from build123d import *

# Parameters (mm, degrees)
SKETCH1_R                  = 2
SCREW_SECTION_DEPTH        = 17
SKETCH2_R                  = 3.5
BAR_SECTION_DEPTH          = 24
MOUNT_SECTION_DEPTH        = 1.6
BAR_TAPER_DEPTH            = 6
MOUNT_FILLET_R             = 0.5
MOUNT_FILLET_OF_MIRROR_2_R = 0.5


with BuildPart() as part:
    # Sketch1 → Screw Section (new body)
    with BuildSketch(Plane.XY):
        Circle(SKETCH1_R)
    screw_section = extrude(amount=SCREW_SECTION_DEPTH)

    # Sketch2 → Bar Section (add)
    with BuildSketch(Plane.XY.offset(17)):
        Circle(SKETCH2_R)
    bar_section = extrude(amount=BAR_SECTION_DEPTH)

    # Sketch3 → Mount Section (add, symmetric)
    with BuildSketch(Plane(origin=(0, 0, 0), x_dir=(1, 0, 0), z_dir=(0, 1, 0))):
        with BuildLine():
            Line((5, -41), (-5, -41))
            Line((-5, -41), (-5, -46))
            ThreePointArc((-5, -46), (0, -51), (5, -46))
            Line((5, -46), (5, -41))
        make_face()
    mount_section = extrude(amount=MOUNT_SECTION_DEPTH, both=True)

    # Sketch4 → Bar Taper (cut, symmetric)
    with BuildSketch(Plane(origin=(0, 0, 0), x_dir=(0, 0, -1), z_dir=(1, 0, 0))):
        Polygon((-36, -3.5), (-41, -1.6), (-41, -3.5), align=None)
        Polygon((-36, 3.5), (-41, 1.6), (-41, 3.5), align=None)
    bar_taper = extrude(amount=BAR_TAPER_DEPTH, both=True, mode=Mode.SUBTRACT)

    # Mount Fillet
    mount_fillet_edges = [part.edges().sort_by_distance(p)[0] for p in [
        (-5, 0, 41),
        (3.401842713, -0.823083322, 41),
        (-3.5, 0, 41),
        (5, 0, 41),
    ]]
    fillet(mount_fillet_edges, radius=MOUNT_FILLET_R)

    # Sketch6 → Ball Hole (revolve, cut)
    with BuildSketch(Plane(origin=(0, 0, 0), x_dir=(0, 0, -1), z_dir=(1, 0, 0))):
        with BuildLine():
            Line((-47.920937271, -1.6), (-46, -1.6))
            Line((-46, -1.6), (-46, 1.6))
            Line((-46, 1.6), (-47.920937271, 1.6))
            ThreePointArc((-47.920937271, 1.6), (-48.5, 0), (-47.920937271, -1.6))
        make_face()
    ball_hole = revolve(axis=Axis((0, -1.6, 46), (0, 1, 0)), mode=Mode.SUBTRACT)

    # Mirror 2: Screw Section, Bar Section, Mount Section, Bar Taper, Ball Hole across Front Plane
    add(screw_section.mirror(Plane.XY))
    add(bar_section.mirror(Plane.XY))
    add(mount_section.mirror(Plane.XY))
    add(bar_taper.mirror(Plane.XY), mode=Mode.SUBTRACT)
    add(ball_hole.mirror(Plane.XY), mode=Mode.SUBTRACT)

    # Mount Fillet of Mirror 2
    mount_fillet_of_mirror_2_edges = [part.edges().sort_by_distance(p)[0] for p in [
        (-5, 0, -41),
        (3.401842713, -0.823083322, -41),
        (-3.5, 0, -41),
        (5, 0, -41),
    ]]
    fillet(mount_fillet_of_mirror_2_edges, radius=MOUNT_FILLET_OF_MIRROR_2_R)


solid = part.part
Geometry: final body of the model. Coordinates: model frame, mm. A direction names the side the tool comes from. Coordinates: 2 decimals unless noted, no trailing zeros. Write each loop counter-clockwise with the first axis right and the second up, starting at its lowest first coordinate (ties: lowest second). Pieces come first, ordered by that corner, then holes. Notation, with made-up numbers: (83.25, 50.5) - (135.25, 50.5) arc R33 cw to (135.25, 82.5) - close; hole circle Ø9 at (-21, -22). An arc over 180 degrees is marked (long way). Return JSON: item names as keys, results as strings.
Item 1: Section query B-B (z = -7). Output: boundary loops of the cut face in (x, y), and give its area (3 significant figures).
Completed:
{"outline": "circle Ø4 at (0, 0)", "area": "12.6 mm2"}
Item 2: Section query C-C (z = -33). Output: boundary loops of the cut face in (x, y).
Completed:
{"outline": "circle Ø7 at (0, 0)"}
Item 3: Line query: L1, parallel to Z at x = 0, y = 0.75; L2, parallel to Z at x = -0.5, y = 1; L3, parallel to Y at x = 4.5, z = -44. Output: solid intervals per line, ascending.
Completed:
{"L1": "z = -51 to -48.38, -43.62 to 43.62, 48.38 to 51", "L2": "z = -50.97 to -48.24, -43.76 to 43.76, 48.24 to 50.97", "L3": "y = -1.6 to 1.6"}
Item 4: Reachability of faces 1 (the face through (0, -2, 0)), 2 (the face through (-0.1, 1.6, 43.7)), 3 (the face through (-0.1, 1.6, -43.7)) from +Z, -Z, +X, -X, +Y, -Y: full face, straight path, thin tool, end or side. Return the list, or none.
Completed:
{"face 1": "none", "face 2": "+Z, +X, -X, +Y", "face 3": "-Z, +X, -X, +Y"}
Item 5: Pin query (flat end, axial travel): pin 1 Ø3 at (x, z) = (3, 38) entering from -Y; pin 2 Ø3 at (x, z) = (-2.5, 44.5) entering from +Y; pin 3 Ø0.9 at (x, y) = (-4, 0.5) entering from +Z. Return the tip coordinate at first contact, or that it passes through.
Completed:
{"pin 1": "stops at y = -3.04", "pin 2": "stops at y = 1.6", "pin 3": "stops at z = 49.52"}
Item 6: Pull-direction query (Z, two-part tool) for faces 4 (the face through (0.051, 2.352, -39.021)), 5 (the face through (2, -2, 17)), 6 (the face through (5, 0, 44)); classes: +Z half, -Z half, draft (parallel to the pull), parting line (faces both ways), or undercut.
Completed:
{"face 4": "-Z half", "face 5": "undercut", "face 6": "draft"}
Item 7: Section query A-A (x = 0). Output: boundary loops of the cut face in (y, z), and give its area (3 significant figures).
Completed:
{"outline": "(-3.5, -36) - (-1.6, -41) - (-1.6, -44.08) arc R2.5 cw to (1.6, -44.08) - (1.6, -41) - (3.5, -36) - (3.5, -17) - (2, -17) - (2, 17) - (3.5, 17) - (3.5, 36) - (1.6, 41) - (1.6, 44.08) arc R2.5 cw to (-1.6, 44.08) - (-1.6, 41) - (-3.5, 36) - (-3.5, 17) - (-2, 17) - (-2, -17) - (-3.5, -17) - close; (-1.6, -51) - (1.6, -51) - (1.6, -47.92) arc R2.5 cw to (-1.6, -47.92) - close; (-1.6, 47.92) arc R2.5 cw to (1.6, 47.92) - (1.6, 51) - (-1.6, 51) - close", "area": "487 mm2"}
